from build123d import *

# Parameters (mm, degrees)
F0_W     = 0.3
F0_H     = 11.95
F0_W_2   = 1.3
F4_DEPTH = 350
F6_DEPTH = 35
F7_SIZE2 = 1
F7_SIZE  = 1


with BuildPart() as f1:
    # F0 (on Front) → F1 (revolve)
    with BuildSketch(Plane.XZ):
        Polygon((-30, 0), (0, 0), (0, 12.5), (-30, 12.5), (-30, 12.225), (-30, 0.275), align=None)
        Polygon((0, 12.5), (0, 0), (360, 0), (360, 12.5), (360, 15), (0, 15), align=None)
        Polygon((360, 12.5), (360, 0), (389, 0), (389, 0.275), (389, 12.225), (389, 12.5), align=None)
        with Locations((-30.15, 6.25)):
            Rectangle(F0_W, F0_H)
        Polygon((-30.3, 0), (-30.3, 0.275), (-30.3, 12.225), (-30.3, 12.5), (-117, 12.5), (-117, 0), align=None)
        with Locations((389.65, 6.25)):
            Rectangle(F0_W_2, F0_H)
        Polygon((390.3, 12.225), (390.3, 0.275), (390.3, 0), (393, 0), (393, 12.5), (390.3, 12.5), align=None)
    revolve(axis=Axis((165, 0, 0), (1, 0, 0)))

    # F3 (on offset) → F4 (cut)
    with BuildSketch(Plane.YZ.offset(355)):
        with BuildLine():
            ThreePointArc((7.4833147735, 13), (0, 15), (-7.4833147735, 13))
            Line((-7.4833147735, 13), (7.4833147735, 13))
        make_face()
        with BuildLine():
            Line((7.4833147735, -13), (-7.4833147735, -13))
            ThreePointArc((-7.4833147735, -13), (0, -15), (7.4833147735, -13))
        make_face()
    extrude(amount=-F4_DEPTH, mode=Mode.SUBTRACT)

    # F5 (on face) → F6 (cut)
    with BuildSketch(Plane(origin=(-117, 0, 0), x_dir=(0, -1, 0), z_dir=(-1, 0, 0))):
        with BuildLine():
            ThreePointArc((6.7823299831, 10.5), (0, 12.5), (-6.7823299831, 10.5))
            Line((-6.7823299831, 10.5), (6.7823299831, 10.5))
        make_face()
        with BuildLine():
            Line((6.7823299831, -10.5), (-6.7823299831, -10.5))
            ThreePointArc((-6.7823299831, -10.5), (0, -12.5), (6.7823299831, -10.5))
        make_face()
    extrude(amount=-F6_DEPTH, mode=Mode.SUBTRACT)

    # F7
    f7_edges = [f1.edges().sort_by_distance(p)[0] for p in [
        (-117, 0, 10.5),
        (-117, 12.5, 0),
        (-117, 0, -10.5),
        (-117, -12.5, 0),
        (393, 0, -12.5),
        (360, 0, -15),
    ]]
    chamfer(f7_edges, length=F7_SIZE, length2=F7_SIZE2)


solid = f1.part
Model file for the job. Use its own axes, mm. A direction names the side the tool comes from. Give positions to 0.01 mm unless a question says otherwise; leave off trailing zeros. Loops run counter-clockwise (first coordinate to the right, second up) from the corner with the lowest first, then second, coordinate; pieces in that order, holes last.
1) Pull direction X, two halves, no side cores. Call faces 4 (the flat face through (182, 0, -13)), 5 (the flat face through (-99, 0, -10.5)), 6 (the flat face through (-117, 0, 0)): +X half, -X half, draft (parallel to the pull), parting line (faces both ways), or undercut.
2) Wall check: line 1 (Y direction, x = 389.8, z = 0) (3 decimals); line 2 (Z direction, x = 196.5, y = 5.75). Give the ranges that are in metal, low to high.
3) Flat gauge pins, fed straight in: pin 1 Ø0.6 at (y, z) = (-3.5, -14) entering from -X; pin 2 Ø2 at (x, z) = (243.5, -11) entering from -Y; pin 3 Ø5 at (x, y) = (-36, 3.5) entering from +Z; pin 4 Ø5 at (y, z) = (7.5, 10) entering from -X. Where does each tip first touch, or does it go through?
4) Saw through at A-A (x = 168.5). Write the cut outline in (y, z), plus the area to 3 significant figures.
5) Tool access for faces 1 (the flat face through (-99, 0, 10.5)), 2 (the flat face through (393, 0, 0)), 3 (the cylindrical face through (391.138, -3.755, 11.923)): list every direction of +Z, -Z, +X, -X, +Y, -Y with a clear straight run to the whole face (end or side of a thin tool).
Answer block:
1. face 4: undercut
1. face 5: draft
1. face 6: -X half
2. line 1: y = -12.225 to -0.275, 0.275 to 12.225
2. line 2: z = -13 to 13
3. pin 1: stops at x = 0
3. pin 2: stops at y = -11.18
3. pin 3: stops at z = 12.46
3. pin 4: stops at x = -117
4. outline: (-7.48, -13) - (7.48, -13) arc R15 ccw to (7.48, 13) - (-7.48, 13) arc R15 ccw to start
4. area: 666 mm2
5. face 1: +Z, -X, +Y, -Y
5. face 2: +Z, -Z, +X, +Y, -Y
5. face 3: +X
